```python
from build123d import *

# Parameters (mm, degrees)
SKETCH1_W           = 100
SKETCH1_H           = 10
BOSS_EXTRUDE1_DEPTH = 10
SKETCH6_W           = 3
SKETCH6_H           = 10
BOSS_EXTRUDE2_DEPTH = 10
SKETCH8_W           = 2
SKETCH8_H           = 10
BOSS_EXTRUDE3_DEPTH = 5
BOSS_EXTRUDE4_DEPTH = 20
SKETCH2_W           = 10
SKETCH2_H           = 5
CUT_EXTRUDE1_DEPTH  = 10
CUT_EXTRUDE2_REACH  = 59.879
SKETCH10_R          = 2.5
CUT_EXTRUDE3_REACH  = 58.789
SKETCH13_R          = 4
SKETCH13_R_2        = 1.25
FILLET1_R           = 3
FILLET2_R           = 3


with BuildPart() as part:
    # Sketch1 → Boss-Extrude1 (new body)
    with BuildSketch(Plane.XY):
        Rectangle(SKETCH1_W, SKETCH1_H)
    extrude(amount=BOSS_EXTRUDE1_DEPTH)

    # Sketch6 → Boss-Extrude2 (add)
    with BuildSketch(Plane(origin=(0, 0, 0), x_dir=(-1, 0, 0), z_dir=(0, 0, -1))):
        with Locations((-23.5, 0)):
            Rectangle(SKETCH6_W, SKETCH6_H)
    boss_extrude2 = extrude(amount=BOSS_EXTRUDE2_DEPTH)

    # Sketch8 → Boss-Extrude3 (add)
    with BuildSketch(Plane.ZY.offset(-22)):
        with Locations((-9, 0)):
            Rectangle(SKETCH8_W, SKETCH8_H)
    boss_extrude3 = extrude(amount=BOSS_EXTRUDE3_DEPTH)

    # Sketch9 → Boss-Extrude4 (add)
    with BuildSketch(Plane.XZ.offset(5)):
        Polygon((17, 2), (17, 0), (22, 0), (22, -8), (17, -8), (17, -10), (25, -10), (25, 0), (25, 2), align=None)
    boss_extrude4 = extrude(amount=BOSS_EXTRUDE4_DEPTH)

    # Mirror3: Boss-Extrude2, Boss-Extrude3, Boss-Extrude4 across plane
    add(boss_extrude2.mirror(Plane(origin=(0, 0, 0), x_dir=(0, 0, 1), z_dir=(1, 0, 0))))
    add(boss_extrude3.mirror(Plane(origin=(0, 0, 0), x_dir=(0, 0, 1), z_dir=(1, 0, 0))))
    add(boss_extrude4.mirror(Plane(origin=(0, 0, 0), x_dir=(0, 0, 1), z_dir=(1, 0, 0))))

    # Sketch2 → Cut-Extrude1 (cut)
    with BuildSketch(Plane(origin=(0, 5, 0), x_dir=(1, 0, 0), z_dir=(0, 1, 0))):
        with Locations((-45, -7.5)):
            Rectangle(SKETCH2_W, SKETCH2_H)
    cut_extrude1 = extrude(amount=-CUT_EXTRUDE1_DEPTH, mode=Mode.SUBTRACT)

    # Mirror4: Cut-Extrude1 across plane
    add(cut_extrude1.mirror(Plane(origin=(0, 0, 0), x_dir=(0, 0, 1), z_dir=(1, 0, 0))), mode=Mode.SUBTRACT)

    # Sketch10 → Cut-Extrude2 (cut, up to next)
    with BuildSketch(Plane.XY.offset(5), mode=Mode.PRIVATE) as cut_extrude2_sk1:
        with Locations((45, 0)):
            Circle(SKETCH10_R)
    cut_extrude2_tool1 = extrude(cut_extrude2_sk1.sketch, amount=-CUT_EXTRUDE2_REACH, mode=Mode.PRIVATE) & part.part
    cut_extrude2 = cut_extrude2_tool1.solids().sort_by_distance((45, 0, 5))[0]
    add(cut_extrude2, mode=Mode.SUBTRACT)

    # Mirror5: Cut-Extrude2 across plane
    add(cut_extrude2.mirror(Plane(origin=(0, 0, 0), x_dir=(0, 0, 1), z_dir=(1, 0, 0))), mode=Mode.SUBTRACT)

    # Sketch13 → Cut-Extrude3 (cut, up to next)
    with BuildSketch(Plane(origin=(0, 0, 0), x_dir=(-1, 0, 0), z_dir=(0, 0, -1)), mode=Mode.PRIVATE) as cut_extrude3_sk1:
        Circle(SKETCH13_R)
    cut_extrude3_tool1 = extrude(cut_extrude3_sk1.sketch, amount=-CUT_EXTRUDE3_REACH, mode=Mode.PRIVATE) & part.part
    # Sketch13 → Cut-Extrude3 (cut, up to next)
    with BuildSketch(Plane(origin=(0, 0, 0), x_dir=(-1, 0, 0), z_dir=(0, 0, -1)), mode=Mode.PRIVATE) as cut_extrude3_sk2:
        with Locations((-7.5, 0)):
            Circle(SKETCH13_R_2)
    cut_extrude3_tool2 = extrude(cut_extrude3_sk2.sketch, amount=-CUT_EXTRUDE3_REACH, mode=Mode.PRIVATE) & part.part
    # Sketch13 → Cut-Extrude3 (cut, up to next)
    with BuildSketch(Plane(origin=(0, 0, 0), x_dir=(-1, 0, 0), z_dir=(0, 0, -1)), mode=Mode.PRIVATE) as cut_extrude3_sk3:
        with Locations((7.5, 0)):
            Circle(SKETCH13_R_2)
    cut_extrude3_tool3 = extrude(cut_extrude3_sk3.sketch, amount=-CUT_EXTRUDE3_REACH, mode=Mode.PRIVATE) & part.part
    add(cut_extrude3_tool1.solids().sort_by_distance((0, 0, 0))[0], mode=Mode.SUBTRACT)
    add(cut_extrude3_tool2.solids().sort_by_distance((7.5, 0, 0))[0], mode=Mode.SUBTRACT)
    add(cut_extrude3_tool3.solids().sort_by_distance((-7.5, 0, 0))[0], mode=Mode.SUBTRACT)

    # Fillet1
    fillet1_edges = [part.edges().sort_by_distance(p)[0] for p in [
        (25, -10, -10),
        (-25, -10, -10),
    ]]
    fillet(fillet1_edges, radius=FILLET1_R)

    # Fillet2
    fillet2_edges = [part.edges().sort_by_distance(p)[0] for p in [
        (-25, -15, 2),
        (25, -15, 2),
    ]]
    fillet(fillet2_edges, radius=FILLET2_R)


solid = part.part
```
The listing builds one solid part. Answer for the finished solid, in the listing's coordinates (mm). A direction names the side the tool comes from. Give positions to 0.01 mm unless a question says otherwise; leave off trailing zeros. Order: outer loops, then holes, each group sorted by start corner. A loop starts at its lowest first (then second) coordinate and runs counter-clockwise, first axis right, second up. Notation, with made-up numbers: (63.5, 40) -> (71.5, 40) arc R15 ccw to (71.5, 62) -> close; hole circle Ø11 at (46.5, 73). An arc over 180 degrees is marked (long way). Answer as CSV lines item,"result". Start each with the question number.
Q1. A cutting plane is placed at A-A (x = -45). Determine the outline of the cut face in (y, z).
Q2. A cutting plane is placed at D-D (z = 3). Determine the outline of the cut face in (x, y).
Q3. A cutting plane is placed at B-B (y = -16.5). Determine the outline of the cut face in (x, z), then the cut area to 3 significant figures.
Q4. Find the intervals of material crossed by L1, parallel to X at y = -0.5, z = -6.75; L2, parallel to Y at x = 7.5, z = 6.5; L3, parallel to Y at x = 0, z = 3.5, in increasing order.
Q5. Which of the six approach directions +Z, -Z, +X, -X, +Y, -Y give full straight-line access (tool end or side, diameter ignored) to faces 4 (the flat face through (-17, -10, -9)), 5 (the flat face through (-20, -15, 2)), 6 (the flat face through (5, -3, 0)), 7 (the flat face through (-47, 2, 5)), 8 (the flat face through (17, -15, 1))?
Q6. Given pin 1 (3 mm diameter, centred on x = -44.5, y = 2, fed in from +Z); pin 2 (2 mm diameter, centred on y = -3, z = 7, fed in from -X); pin 3 (2 mm diameter, centred on y = -5, z = -9, fed in from -X); pin 4 (3 mm diameter, centred on x = 23.5, z = 3, fed in from -Y), each flat-ended and moving along its own axis, determine where each tip first touches the part or whether it passes through.
Q7. Determine the mould class of faces 1 (the flat face through (20, -15, 2)), 2 (the flat face through (23, -25, -4)), 3 (the cylindrical face through (47.31, -0.96, 2.54)) for opening direction Y: pulls with the +Y half, pulls with the -Y half, needs draft (parallel to the pull), parting line crosses it, or undercut.
Q8. A cutting plane is placed at C-C (z = -3.25). Determine the outline of the cut face in (x, y), then the cut area to 3 significant figures.
Results found:
1,outline,"(-5, 0) -> (-2.5, 0) -> (-2.5, 5) -> (-5, 5) -> close; (2.5, 0) -> (5, 0) -> (5, 5) -> (2.5, 5) -> close"
2,outline,"(-50, -5) -> (50, -5) -> (50, 5) -> (-50, 5) -> close; hole circle Ø5 at (-45, 0); hole circle Ø2.5 at (-7.5, 0); hole circle Ø8 at (0, 0); hole circle Ø2.5 at (7.5, 0); hole circle Ø5 at (45, 0)"
3,outline,"(-25, -7) arc R3 ccw to (-22, -10) -> (-17, -10) -> (-17, -8) -> (-22, -8) -> (-22, 0) -> (-17, 0) -> (-17, 2) -> (-22, 2) arc R3 ccw to (-25, -1) -> close; (17, -10) -> (22, -10) arc R3 ccw to (25, -7) -> (25, -1) arc R3 ccw to (22, 2) -> (17, 2) -> (17, 0) -> (22, 0) -> (22, -8) -> (17, -8) -> close"
3,area,"104 mm2"
4,L1,"-25 to -22, 22 to 25"
4,L2,"-5 to -1.25, 1.25 to 5"
4,L3,"-5 to -4, 4 to 5"
5,face 4,"-Z, +Y, -Y"
5,face 5,"+Z, +X, -X, -Y"
5,face 6,"+Y, -Y"
5,face 7,"+Z, -X, +Y, -Y"
5,face 8,"+Z, -Z, -Y"
6,pin 1,"z = 5"
6,pin 2,"x = -40"
6,pin 3,"x = -24.83"
6,pin 4,"y = -25"
7,face 1,"needs draft"
7,face 2,"pulls with the -Y half"
7,face 3,"undercut"
8,outline,"(-25, -25) -> (-22, -25) -> (-22, 5) -> (-25, 5) -> close; (22, -25) -> (25, -25) -> (25, 5) -> (22, 5) -> close"
8,area,"180 mm2"
